from build123d import *

# Parameters (mm, degrees)
SKETCH_1_R      = 1.5
EXTRUDE_1_DEPTH = 5


with BuildPart() as part:
    # 스케치1 → 보스-돌출1 (new body)
    with BuildSketch(Plane(origin=(0, 0, 0), x_dir=(1, 0, 0), z_dir=(0, 1, 0))):
        Polygon((45.770598642, -110.5), (110.5, -45.770598642), (110.5, 45.770598642), (45.770598642, 110.5), (-45.770598642, 110.5), (-110.5, 45.770598642), (-110.5, -45.770598642), (-45.770598642, -110.5), align=None)
        with Locations((-5, 105.5)):
            Circle(SKETCH_1_R, mode=Mode.SUBTRACT)
        with Locations((-5, 95.5)):
            Circle(SKETCH_1_R, mode=Mode.SUBTRACT)
        with Locations((5, 95.5)):
            Circle(SKETCH_1_R, mode=Mode.SUBTRACT)
        with Locations((5, 105.5)):
            Circle(SKETCH_1_R, mode=Mode.SUBTRACT)
        with Locations((105.5, 5)):
            Circle(SKETCH_1_R, mode=Mode.SUBTRACT)
        with Locations((95.5, 5)):
            Circle(SKETCH_1_R, mode=Mode.SUBTRACT)
        with Locations((95.5, -5)):
            Circle(SKETCH_1_R, mode=Mode.SUBTRACT)
        with Locations((105.5, -5)):
            Circle(SKETCH_1_R, mode=Mode.SUBTRACT)
        with Locations((5, -105.5)):
            Circle(SKETCH_1_R, mode=Mode.SUBTRACT)
        with Locations((5, -95.5)):
            Circle(SKETCH_1_R, mode=Mode.SUBTRACT)
        with Locations((-5, -95.5)):
            Circle(SKETCH_1_R, mode=Mode.SUBTRACT)
        with Locations((-5, -105.5)):
            Circle(SKETCH_1_R, mode=Mode.SUBTRACT)
        with Locations((-105.5, -5)):
            Circle(SKETCH_1_R, mode=Mode.SUBTRACT)
        with Locations((-95.5, -5)):
            Circle(SKETCH_1_R, mode=Mode.SUBTRACT)
        with Locations((-95.5, 5)):
            Circle(SKETCH_1_R, mode=Mode.SUBTRACT)
        with Locations((-105.5, 5)):
            Circle(SKETCH_1_R, mode=Mode.SUBTRACT)
    extrude(amount=EXTRUDE_1_DEPTH)


solid = part.part
Can you work these out from the model? Positions are in its coordinate system, mm. Coordinates: 2 decimals unless noted, no trailing zeros. Loops run counter-clockwise (first coordinate to the right, second up) from the corner with the lowest first, then second, coordinate; pieces in that order, holes last. Notation, with made-up numbers: M 45.25,-20.5 L 54.25,-20.5 A18 cw 54.25,4.5 Z; hole C 20,-5 d4. An arc over 180 degrees is marked long. Return JSON: item names as keys, results as strings. Group by question number.
Item 1: Imagine slicing it at A-A (y = 3.45). Give the number of separate pieces and of enclosed holes in the cut face, and give its area (3 significant figures).
Item 2: Imagine slicing it at B-B (z = -81.5). Please give me the cut outline in (x, y), and give its area (3 significant figures).
Item 3: Imagine slicing it at C-C (x = 91). Please give me the cut outline in (y, z).
Item 4: I'm going to push flat-ended pins straight in: pin 1 Ø3 at (y, z) = (2.5, 69) entering from -X; pin 2 Ø4 at (x, z) = (5, -95.5) entering from -Y. Where does each tip first touch, or does it pass through?
Item 5: If I drill on L1, parallel to Z at x = -5, y = 2.25; L2, parallel to Z at x = -95.5, y = 2, over which ranges is the centre line in solid material (lowest first)? Write a range as from..to.
Verdict:
{
 "1": {"separate pieces": "1", "enclosed holes": "16", "area": "40,300 mm^2"},
 "2": {"outline": "M -74.77,0 L 74.77,0 L 74.77,5 L -74.77,5 Z", "area": "748 mm^2"},
 "3": {"outline": "M 0,-65.27 L 5,-65.27 L 5,65.27 L 0,65.27 Z"},
 "4": {"pin 1": "stops at x = -88.77", "pin 2": "stops at y = 0"},
 "5": {"L1": "z = -110.5..-107, -104..-97, -94..94, 97..104, 107..110.5", "L2": "z = -60.77..-6.5, -3.5..3.5, 6.5..60.77"}
}
